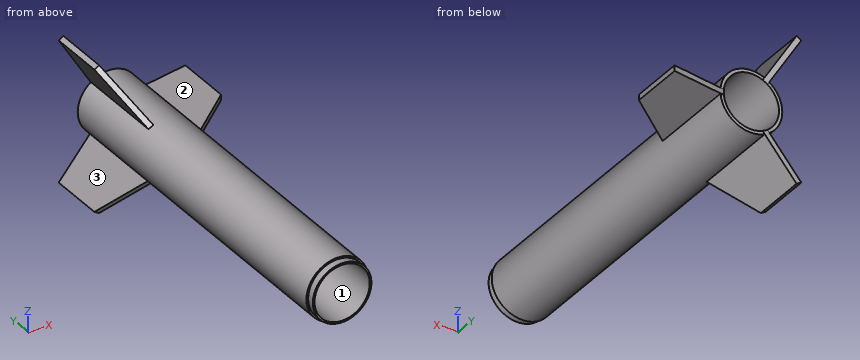
Autodesk Inventor part; units mm, degrees
ref_plane "YZ Plane" through (0, 0, 0) normal (1, 0, 0) x (0, 1, 0)
ref_plane "XZ Plane" through (0, 0, 0) normal (0, 1, 0) x (-1, 0, 0)
ref_plane "XY Plane" through (0, 0, 0) normal (0, 0, 1) x (1, 0, 0)
sketch "Sketch1" plane through (0, 0, 0) normal (0, 1, 0) x (-1, 0, 0)
  circle A0 centre (0, 0) radius 15
  circle A1 centre (0, 0) radius 15.9
  circle A2 centre (0, 0) radius 16.8
  dimension "d0" = 30
  dimension "d1" = 31.8
  dimension "d2" = 33.6
extrude "Extrusion1" add sketch "Sketch1" along normal blind 96 and the other way blind 100 contours A1
extrude "Extrusion2" add sketch "Sketch1" along normal blind 96 and the other way blind 96 contours A2
sketch "Sketch4" plane through (0, 0, 0) normal (0, 0, 1) x (1, 0, 0)
  line L0 (45, 99.9302) -> (45, 71.173)
  line L1 (45, 71.173) -> (15, 46)
  line L2 (15, 46) -> (15, 96)
  line L3 (15, 96) -> (45, 101.173)
  line L4 (45, 101.173) -> (45, 99.9302)
  line L5 (-15, 96) -> (15, 96)
  line L6 (16.8, 96) -> (-16.8, 96)
  line L7 (-15, 96) -> (15, 96)
  line L8 (15.9, -100) -> (15, -100)
  line L9 (15, -100) -> (15, 96)
  line L10 (15, 96) -> (16.8, 96)
  line L11 (16.8, 96) -> (16.8, -96)
  line L12 (16.8, -96) -> (15.9, -96)
  line L13 (-15, -100) -> (-15.9, -100)
  line L14 (-16.8, -96) -> (-16.8, 96)
  line L15 (-16.8, 96) -> (-15, 96)
  line L16 (-15, 96) -> (-15, -100)
  line L17 (-15.9, -96) -> (-16.8, -96)
  line L18 (15.9, -96) -> (15.9, -100)
  line L19 (-15.9, -100) -> (-15.9, -96)
  point P0 (0, 0)
  point P1 (16.8, 47.5104)
  dimension "d18" = 50
  dimension "d21" = 50
  dimension "d24" = 30
  dimension "d25" = 30
extrude "Extrusion4" add sketch "Sketch4" along normal mid plane 3 contours L0 L1 L11 L6 L3 L4
pattern_circular "Circular Pattern2" count 3 over 360 about axis through (0, -10, 0) along (0, 1, 0) of "Extrusion4"
properties part number "tail" material "ABS Plastic"
Geometry check sheet. Reference: the model listing, model coordinates, mm. Face numbers are marked on the shaded views. Round coordinates to 2 decimals unless told otherwise and drop trailing zeros. Write each loop counter-clockwise with the first axis right and the second up, starting at its lowest first coordinate (ties: lowest second). Pieces come first, ordered by that corner, then holes. Notation, with made-up numbers: (80, 9.5) -> (102, 9.5) arc R6 ccw to (102, 20.5) -> close; hole circle Ø1 at (23, 78). An arc over 180 degrees is marked (long way). One line per item, written item: value. Start each with the question number.
(1) Cross-section at A-A, the plane y = 77.5. Record the cut outline in (x, z), and give its area (3 significant figures).
(2) Draft check along X on the marked faces 1, 2 and 3. Enter one of: +X half, -X half, draft (parallel to the pull), parting line (faces both ways), or undercut.
(3) Cross-section at B-B, the plane x = 0. Record the cut outline in (y, z).
(4) Cross-section at D-D, the plane y = 56. Record the cut outline in (x, z), and give its area (3 significant figures).
(5) Scan lines: line 1 (X direction, y = 25.5, z = 0); line 2 (Y direction, x = -2, z = -15). Record each from-to range of solid material in increasing order. Write a range as [from, to].
(6) Go/stop test with flat-tipped pins: pin 1 Ø8 at (x, y) = (15, 25) entering from +Z; pin 2 Ø10 at (y, z) = (-6.5, -18) entering from -X; pin 3 Ø10 at (x, z) = (-12, 2.5) entering from +Y. Record where each tip stops, or that it passes through.
(7) Cross-section at C-C, the plane y = -54. Record the cut outline in (x, z).
Answer:
1. outline: (-23.8, -38.22) -> (-21.2, -39.72) -> (-7.1, -15.3) -> (-9.7, -13.8) -> close; (-23.8, 38.22) -> (-9.7, 13.8) -> (-7.1, 15.3) -> (-21.2, 39.72) -> close; circle Ø33.6 at (0, 0); (16.8, -1.5) -> (45, -1.5) -> (45, 1.5) -> (16.8, 1.5) -> close; hole circle Ø30 at (0, 0)
1. area: 434 mm²
2. face 1: undercut
2. face 2: draft
2. face 3: -X half
3. outline: (-100, -15.9) -> (-96, -15.9) -> (-96, -16.8) -> (96, -16.8) -> (96, -15) -> (-100, -15) -> close; (-100, 15) -> (96, 15) -> (96, 16.8) -> (-96, 16.8) -> (-96, 15.9) -> (-100, 15.9) -> close
4. outline: circle Ø33.6 at (0, 0); (-14.76, -22.56) -> (-12.16, -24.06) -> (-7.1, -15.3) -> (-9.7, -13.8) -> close; (-14.76, 22.56) -> (-9.7, 13.8) -> (-7.1, 15.3) -> (-12.16, 24.06) -> close; (16.8, -1.5) -> (26.92, -1.5) -> (26.92, 1.5) -> (16.8, 1.5) -> close; hole circle Ø30 at (0, 0)
4. area: 271 mm²
5. line 1: [-16.8, -15], [15, 16.8]
5. line 2: [-100, 96]
6. pin 1: z = 12.7
6. pin 2: x = -10.64
6. pin 3: y = 96
7. outline: circle Ø33.6 at (0, 0); hole circle Ø30 at (0, 0)
